```python
from build123d import *

# Parameters (mm, degrees)
SKETCH005_W       = 20
SKETCH005_H       = 40
SKETCH005_R       = 1.3
PAD002_DEPTH      = 5
SKETCH006_R       = 2.5
PAD003_DEPTH      = 20
SKETCH007_R       = 1.6
POCKET003_DEPTH   = 0.5
POCKET003_FACE4_W = 40
POCKET003_FACE4_H = 20
POCKET003_FACE4_R = 1.3
POCKET006_DEPTH   = 3
SKETCH014_R       = 1.3
POCKET009_DEPTH   = 5
SKETCH016_R       = 3
SKETCH016_R_2     = 2.5
PAD008_DEPTH      = 20
SKETCH017_R       = 1.375
POCKET010_DEPTH   = 5


with BuildPart() as part:
    # Sketch005 (on DatumPlane) → Pad002 (new body)
    with BuildSketch(Plane(origin=(0, 0, 20), x_dir=(0, 0, -1), z_dir=(-1, 0, 0))):
        with Locations((10, 20)):
            Rectangle(SKETCH005_W, SKETCH005_H)
        with Locations((10, 30)):
            Circle(SKETCH005_R, mode=Mode.SUBTRACT)
        with Locations((10, 10)):
            Circle(SKETCH005_R, mode=Mode.SUBTRACT)
    extrude(amount=PAD002_DEPTH)

    # Sketch006 (on Face8 of Pad002) → Pad003 (join)
    with BuildSketch(Plane(origin=(-5, 0, 20), x_dir=(0, 0, -1), z_dir=(-1, 0, 0))):
        with Locations((10, 30)):
            Circle(SKETCH006_R)
        with Locations((10, 10)):
            Circle(SKETCH006_R)
    extrude(amount=PAD003_DEPTH)

    # Sketch007 → Pocket003 (cut)
    with BuildSketch(Plane(origin=(-5, 0, 20), x_dir=(0, 0, -1), z_dir=(-1, 0, 0))):
        with Locations((10, 20)):
            Circle(SKETCH007_R)
    extrude(amount=-POCKET003_DEPTH, mode=Mode.SUBTRACT)

    # Pocket003 Face4 → Pocket006 (cut)
    with BuildSketch(Plane(origin=(0, -20, 10), x_dir=(0, -1, 0), z_dir=(1, 0, 0))):
        Rectangle(POCKET003_FACE4_W, POCKET003_FACE4_H)
        with Locations((10, 0)):
            Circle(POCKET003_FACE4_R, mode=Mode.SUBTRACT)
        with Locations((-10, 0)):
            Circle(POCKET003_FACE4_R, mode=Mode.SUBTRACT)
    extrude(amount=-POCKET006_DEPTH, mode=Mode.SUBTRACT)

    # Sketch014 (on Face14 of Pocket006) → Pocket009 (cut)
    with BuildSketch(Plane(origin=(-25, 0, 20), x_dir=(0, 0, -1), z_dir=(-1, 0, 0))):
        with Locations((10, 10)):
            Circle(SKETCH014_R)
        with Locations((10, 30)):
            Circle(SKETCH014_R)
    extrude(amount=-POCKET009_DEPTH, mode=Mode.SUBTRACT)

    # Sketch016 (on Face14 of Pocket009) → Pad008 (join)
    with BuildSketch(Plane(origin=(-25, 0, 20), x_dir=(0, 0, -1), z_dir=(-1, 0, 0))):
        with Locations((10, 30)):
            Circle(SKETCH016_R)
        with Locations((10, 30)):
            Circle(SKETCH016_R_2, mode=Mode.SUBTRACT)
        with Locations((10, 10)):
            Circle(SKETCH016_R)
        with Locations((10, 10)):
            Circle(SKETCH016_R_2, mode=Mode.SUBTRACT)
    extrude(amount=-PAD008_DEPTH)

    # Sketch017 (on Face15 of Pad008) → Pocket010 (cut)
    with BuildSketch(Plane(origin=(-25, 0, 20), x_dir=(0, 0, -1), z_dir=(-1, 0, 0))):
        with Locations((10, 30)):
            Circle(SKETCH017_R)
        with Locations((10, 10)):
            Circle(SKETCH017_R)
    extrude(amount=-POCKET010_DEPTH, mode=Mode.SUBTRACT)


with BuildPart() as part_1:
    # Body002 placement: moved
    add(part.part.moved(Location((-20, 0, 0))))


solid = part_1.part
```
Geometry: final body of the model. Coordinates: model frame, mm. A direction names the side the tool comes from. Coordinates: 2 decimals unless noted, no trailing zeros. Order: outer loops, then holes, each group sorted by start corner. A loop starts at its lowest first (then second) coordinate and runs counter-clockwise, first axis right, second up. Notation, with made-up numbers: M -39,33 L -10,33 A22 cw -10,47 Z; hole C 64.25,9 d6. An arc over 180 degrees is marked long. Answer in a Markdown table with one row per item. Add a question column.
Q1. Reachability of faces 1 (the flat face through (-24, -40, 10)), 2 (the cylindrical face through (-35.14, -32.03, 12.21)), 3 (the flat face through (-25, -10, 10)) from +Z, -Z, +X, -X, +Y, -Y: full face, straight path, thin tool, end or side. Return the list, or none.
Q2. Section query C-C on x = -43. Return the cut outline in (y, z) (3 decimals).
Q3. Section query D-D on x = -35.5. Return the cut outline in (y, z).
Q4. Section query B-B on y = -20. Return the cut outline in (x, z).
Q5. Line query: L1, parallel to Y at x = -43.45, z = 10 (3 decimals); L2, parallel to Z at x = -42.9, y = -10 (3 decimals); L3, parallel to Y at x = -24.8, z = 10. Output: solid intervals per line, ascending.
Q6. Contact query for flat-ended pins moving along their axis: P1, Ø8, axis at x = -31, z = 5.5, coming from the +Y side; P2, Ø2, axis at y = -10, z = 10, coming from the -X side; P3, Ø2.5, axis at y = -30, z = 10, coming from the +X side. Output: stop coordinate, or through.
Q7. Mould query, pull axis Y, two halves, no side actions, for faces 4 (the cylindrical face through (-23.99, -10.39, 8.76)), 5 (the flat face through (-24, 0, 10)), 6 (the flat face through (-24, -20, 20)), 7 (the flat face through (-24.5, -20, 10)). Classes: released by +Y, released by -Y, zero draft, split by the parting line, or undercut.
Completed:
| question | item | result |
|---|---|---|
| 1 | face 1 | +Z, -Z, +X, -X, -Y |
| 1 | face 2 | -X |
| 1 | face 3 | +X |
| 2 | outline | C -30,10 d6; C -10,10 d6; hole C -30,10 d2.75; hole C -10,10 d2.75 |
| 3 | outline | C -30,10 d6; C -10,10 d6 |
| 4 | outline | M -25,0 L -23,0 L -23,20 L -25,20 L -25,11.6 L -24.5,11.6 L -24.5,8.4 L -25,8.4 Z |
| 5 | L1 | y = -33 to -31.375, -28.625 to -27, -13 to -11.375, -8.625 to -7 |
| 5 | L2 | z = 7 to 8.625, 11.375 to 13 |
| 5 | L3 | y = -40 to -31.3, -28.7 to -21.6, -18.4 to -11.3, -8.7 to 0 |
| 6 | P1 | stops at y = -7.04 |
| 6 | P2 | stops at x = -40 |
| 6 | P3 | stops at x = -25 |
| 7 | face 4 | undercut |
| 7 | face 5 | released by +Y |
| 7 | face 6 | zero draft |
| 7 | face 7 | undercut |
